from build123d import *

# Parameters (mm, degrees)
F1_DEPTH      = 15
F1_DEPTH_BACK = 20
F2_R          = 2
F3_DEPTH      = 14.7596476454
F4_R          = 0.99999
F5_SIZE2      = 7.2794046853
F5_SIZE       = 20
F6_SIZE       = 6
F7_T1_DEPTH   = 20.4974746831
F7_T3_DEPTH   = 30.5072638373
F7_T5_DEPTH   = 12.1714443248


# Not quite as in the source:
# - a fillet or chamfer that OpenCascade refuses, or shapes differently, is made with other operations: its cross-section is extruded or revolved along the edge and cut away or added
# - a fillet or chamfer is up to 0.001 mm smaller than in the source, because OpenCascade refuses the exact size
# - a feature names something its author has since deleted; it is built from what else it names


with BuildPart() as f1:
    # F0 (on Top) → F1 (new body, two sides)
    with BuildSketch(Plane.XY) as f1_sk:
        with BuildLine():
            Line((0, 10), (0, 0))
            Line((0, 0), (6, 0))
            Line((6, 0), (6, 10))
            ThreePointArc((6, 10), (3, 9.4529868603), (0, 10))
        make_face()
        with BuildLine():
            ThreePointArc((11.5, 17.9529868603), (9.9910657271, 13.1182169588), (6, 10))
            Line((6, 10), (14.7586476454, 10))
            Line((14.7586476454, 10), (11.0298702995, 20.7406710197))
            ThreePointArc((11.0298702995, 20.7406710197), (11.3816435604, 19.3665112594), (11.5, 17.9529868603))
        make_face()
        with BuildLine():
            ThreePointArc((5.9635743738, 25.9196189549), (-4.9598303138, 20.9347818526), (0, 10))
            ThreePointArc((0, 10), (3, 9.4529868603), (6, 10))
            ThreePointArc((6, 10), (9.9910657271, 13.1182169588), (11.5, 17.9529868603))
            ThreePointArc((11.5, 17.9529868603), (11.3816435604, 19.3665112594), (11.0298702995, 20.7406710197))
            ThreePointArc((11.0298702995, 20.7406710197), (10.6165760284, 21.7262837746), (10.0828666254, 22.6522421594))
            Line((10.0828666254, 22.6522421594), (8.4163097724, 21.5465350302))
            ThreePointArc((8.4163097724, 21.5465350302), (9.2231830087, 19.8296842892), (9.5, 17.9529868603))
            ThreePointArc((9.5, 17.9529868603), (-1.83621149, 13.6100548526), (3.6965974081, 24.4155522991))
            Line((3.6965974081, 24.4155522991), (5.9635743738, 25.9196189549))
        make_face()
    extrude(amount=F1_DEPTH)
    extrude(f1_sk.sketch, amount=-F1_DEPTH_BACK)

    # F2 (on face) → F3 (cut, through all)
    with BuildSketch(Plane(origin=(0, 0, 0), x_dir=(0, -1, 0), z_dir=(-1, 0, 0))):
        with Locations((-5, 5)):
            Circle(F2_R)
    extrude(amount=-F3_DEPTH, mode=Mode.SUBTRACT)

    # F4 (radius 1 in the source; OpenCascade refuses exactly that, so slightly less here)
    f4_edges = [f1.edges().sort_by_distance(p)[0] for p in [
        (5.963574, 25.919619, -2.5),
        (8.41631, 21.546535, -2.5),
        (10.082867, 22.652242, -2.5),
    ]]
    fillet(f4_edges, radius=F4_R)

    # F5
    f5_edges = [f1.edges().sort_by_distance(p)[0] for p in [
        (3, 0, -20),
    ]]
    f5_side = f1.faces().sort_by_distance((3, 0, -2.5))[0]
    chamfer(f5_edges, length=F5_SIZE, length2=F5_SIZE2, reference=f5_side)

    # F6
    f6_edges = [f1.edges().sort_by_distance(p)[0] for p in [
        (3, 0, 15),
    ]]
    chamfer(f6_edges, length=F6_SIZE)

    # F7: fillet of radius 7 on 4 edges, made by hand

    # F7_s2 → F7_t1 (cut)
    with BuildSketch(Plane.YZ.offset(-7.2487373415)):
        with BuildLine():
            ThreePointArc((0, 6.1005050634), (0.5328432724, 8.7792890899), (2.0502525317, 11.0502525317))
            Line((2.0502525317, 11.0502525317), (0, 9))
            Line((0, 9), (0, 6.1005050634))
        make_face()
        with BuildLine():
            ThreePointArc((3.9497474683, 12.9497474683), (6.2207109101, 14.4671567276), (8.8994949366, 15))
            Line((8.8994949366, 15), (6, 15))
            Line((6, 15), (3.9497474683, 12.9497474683))
        make_face()
    extrude(amount=F7_T1_DEPTH, mode=Mode.SUBTRACT)

    # F7_s4 → F7_t3 (cut)
    with BuildSketch(Plane.YZ.offset(-12.2536319187)):
        with BuildLine():
            ThreePointArc((5.6030091073, -15.3941410033), (8.1658223983, -18.73406431), (12.1808574528, -20))
            Line((12.1808574528, -20), (7.2794046853, -20))
            Line((7.2794046853, -20), (5.6030091073, -15.3941410033))
        make_face()
    extrude(amount=F7_T3_DEPTH, mode=Mode.SUBTRACT)

    # F7_s6 → F7_t5 (cut)
    with BuildSketch(Plane.YZ.offset(-3.0857221624)):
        with BuildLine():
            ThreePointArc((0, 1.234288865), (0.1063457289, 0.0187516213), (0.4221516545, -1.1598521383))
            Line((0.4221516545, -1.1598521383), (0, 0))
            Line((0, 0), (0, 1.234288865))
        make_face()
    extrude(amount=F7_T5_DEPTH, mode=Mode.SUBTRACT)


solid = f1.part
Read the model definition and answer for the solid it produces. Units are mm, in the model's axes. A direction names the side the tool comes from. Give positions to 0.01 mm unless a question says otherwise; leave off trailing zeros. Write each loop counter-clockwise with the first axis right and the second up, starting at its lowest first coordinate (ties: lowest second). Pieces come first, ordered by that corner, then holes. Notation, with made-up numbers: (84.25, 80) - (113.25, 80) arc R12 cw to (113.25, 103) - close; hole circle Ø6 at (32.5, -28.5). An arc over 180 degrees is marked (long way). Answer in a Markdown table with one row per item. Add a question column.
Item 1: Find the intervals of material crossed by L1, parallel to Y at x = 1.25, z = -3.5; L2, parallel to Y at x = 3, z = -9; L3, parallel to X at y = 14.5, z = -3.5, in increasing order.
Item 2: A tool of negligible diameter and unlimited length cuts with its end or side. For faces 1 (the face through (8.785, 21.502, -2.255)), 2 (the face through (0, 6, -2)), 3 (the face through (6, 6, -2)), 4 (the face through (11, 16, -20)), 5 (the face through (2.96, 3.05, -8.38)), from which of +Z, -Z, +X, -X, +Y, -Y can it reach the whole face along a straight path? Write none if from no direction.
Item 3: Flat-ended cylindrical pins translate along their axes: P1, Ø6, axis at x = 2, y = 22, coming from the +Z side; P2, Ø12, axis at y = 10.5, z = 7, coming from the -X side; P3, Ø5, axis at y = 5, z = 0.5, coming from the -X side; P4, Ø1.5, axis at x = -2.5, y = 7.5, coming from the +Z side. Find the tip coordinate at first contact, or state that the pin passes through.
Item 4: Determine the mould class of faces 6 (the face through (6.833, 12.516, 15)), 7 (the face through (10, 10, -2)), 8 (the face through (-3.5, 19.9, -20)), 9 (the face through (3, 7, 5)) for opening direction Z: pulls with the +Z half, pulls with the -Z half, needs draft (parallel to the pull), parting line crosses it, or undercut.
Item 5: Section D-D, the plane x = -1.75 is taken. Write down the section's boundary in (y, z), and give its area (3 significant figures).
Item 6: Section C-C, the plane y = 5 is taken. Write down the section's boundary in (x, z).
Item 7: Section A-A, the plane x = 3 is taken. Write down the section's boundary in (y, z), and give its area (3 significant figures).
Recorded:
| question | item | result |
|---|---|---|
| 1 | L1 | y = 1.27 to 11.69, 24.21 to 26.27 |
| 1 | L2 | y = 3.28 to 11.45, 24.45 to 26.45 |
| 1 | L3 | x = -4.77 to -2.51, 8.51 to 13.2 |
| 2 | face 1 | +Z, -Z |
| 2 | face 2 | +Z, -Z, -X, -Y |
| 2 | face 3 | +Z, -Z, +X, -Y |
| 2 | face 4 | -Z, +X, -X, +Y, -Y |
| 2 | face 5 | -Z, +X, -X, -Y |
| 3 | P1 | stops at z = 15 |
| 3 | P2 | stops at x = -5.37 |
| 3 | P3 | stops at x = 0 |
| 3 | P4 | passes through |
| 4 | face 6 | pulls with the +Z half |
| 4 | face 7 | needs draft |
| 4 | face 8 | pulls with the -Z half |
| 4 | face 9 | undercut |
| 5 | outline | (10.9, -19.88) arc R7 ccw to (12.18, -20) - (13.52, -20) - (13.52, 15) - (10.9, 15) - close; (22.39, -20) - (25, -20) - (25, 15) - (22.39, 15) - close |
| 5 | area | 183 mm2 |
| 6 | outline | (0, -13.74) - (6, -13.74) - (6, 3) - (0, 3) - close; (0, 7) - (6, 7) - (6, 13.81) - (0, 13.81) - close |
| 7 | outline | (0, 1.23) arc R7 ccw to (0.42, -1.16) - (5.6, -15.39) arc R7 ccw to (11.45, -19.96) - (11.45, 15) - (8.9, 15) arc R7 ccw to (3.95, 12.95) - (2.05, 11.05) arc R7 ccw to (0, 6.1) - close; (24.45, -20) - (26.45, -20) - (26.45, 15) - (24.45, 15) - close; hole circle Ø4 at (5, 5) |
| 7 | area | 361 mm2 |
